Design review of the part built by this model. Coordinates are the model's own, in mm. Face numbers are marked on the shaded views. A direction names the side the tool comes from. Round coordinates to 2 decimals unless told otherwise and drop trailing zeros. Loops run counter-clockwise (first coordinate to the right, second up) from the corner with the lowest first, then second, coordinate; pieces in that order, holes last. Notation, with made-up numbers: (78.5, 12.25) - (84.5, 12.25) arc R24 ccw to (84.5, 22.25) - close; hole circle Ø1 at (0, -28). An arc over 180 degrees is marked (long way). Return JSON: item names as keys, results as strings. Group by question number.
(1) Clearance check with flat-ended pins moving along their axes: pin 1 (3 mm diameter, centred on x = -43.5, z = 25.5, fed in from -Y); pin 2 (3 mm diameter, centred on x = -41, z = 31.5, fed in from -Y); pin 3 (2 mm diameter, centred on x = -45.5, y = 3.5, fed in from -Z). State where each tip first meets the part, or that it passes through.
(2) We need section B-B, the plane z = 16. Write out the cut boundary in (x, y) (3 decimals), and give its area (3 significant figures).
(3) Wall thickness on L1, parallel to X at y = 0.5, z = 12.25; L2, parallel to X at y = 2.25, z = 14.75; L3, parallel to Y at x = -42.5, z = 23: over which ranges is each line inside the solid? List them lowest first. Write a range as [from, to].
(4) For the marked faces 1, 2 and 3, list the 3-axis set-ups (+Z, -Z, +X, -X, +Y, -Y) from which the entire face can be reached by the end or side of a thin tool; tool diameter is ignored.
(5) We need section A-A, the plane z = 19. Write out the cut boundary in (x, y), and give its area (3 significant figures).
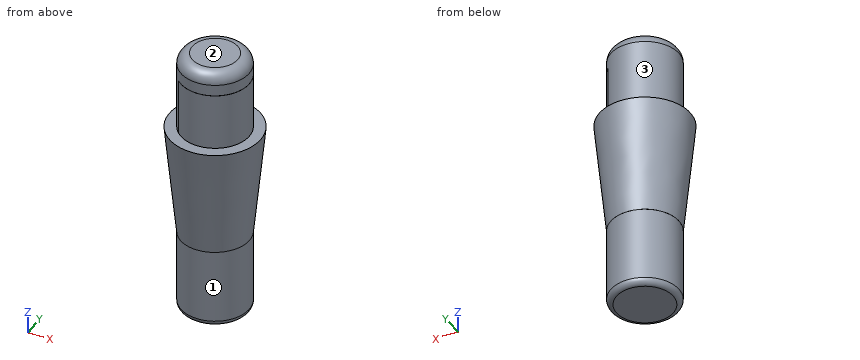
from build123d import *

# Parameters (mm, degrees)
CYLINDER_R        = 3
CYLINDER_DEPTH    = 22
FILLET002_R       = 0.5
CYLINDER001_R     = 3
CYLINDER001_DEPTH = 7
FILLET001_R       = 1


with BuildPart() as fillet002:
    # Cylinder → Cylinder (new body)
    with BuildSketch(Plane(origin=(-43.635, 0.385, 10.17), x_dir=(1, 0, 0), z_dir=(0, 0, 1))):
        Circle(CYLINDER_R)
    extrude(amount=CYLINDER_DEPTH)

    # Fillet002
    fillet002_edges = [fillet002.edges().sort_by_distance(p)[0] for p in [
        (-46.635, 0.385, 10.17),
    ]]
    fillet(fillet002_edges, radius=FILLET002_R)


with BuildPart() as cone:
    # Cone → Cone (revolve)
    with BuildSketch(Plane(origin=(-43.64, 0.39, 17.17), x_dir=(1, 0, 0), z_dir=(0, -1, 0))):
        Polygon((0, 0), (3, 0), (4, 10), (0, 10), align=None)
    revolve(axis=Axis((-43.64, 0.39, 17.17), (0, 0, 1)))


with BuildPart() as fusion001:
    # Cylinder001 → Cylinder001 (new body)
    with BuildSketch(Plane(origin=(-43.64, 0.39, 27.17), x_dir=(1, 0, 0), z_dir=(0, 0, 1))):
        Circle(CYLINDER001_R)
    extrude(amount=CYLINDER001_DEPTH)

    # Fillet001
    fillet001_edges = [fusion001.edges().sort_by_distance(p)[0] for p in [
        (-46.64, 0.39, 34.17),
    ]]
    fillet(fillet001_edges, radius=FILLET001_R)

    # Fusion001: union Fillet002, Cone
    add(fillet002.part)
    add(cone.part)


solid = fusion001.part
Solutions:
{
 "1": {"pin 1": "y = -3.59", "pin 2": "y = -2.39", "pin 3": "z = 10.19"},
 "2": {"outline": "circle Ø6 at (-43.635, 0.385)", "area": "28.3 mm^2"},
 "3": {"L1": "[-46.63, -40.64]", "L2": "[-45.98, -41.29]", "L3": "[-3.01, 3.79]"},
 "4": {"face 1": "-Z", "face 2": "+Z, +X, -X, +Y, -Y", "face 3": "+Z"},
 "5": {"outline": "circle Ø6.37 at (-43.64, 0.39)", "area": "31.8 mm^2"}
}
